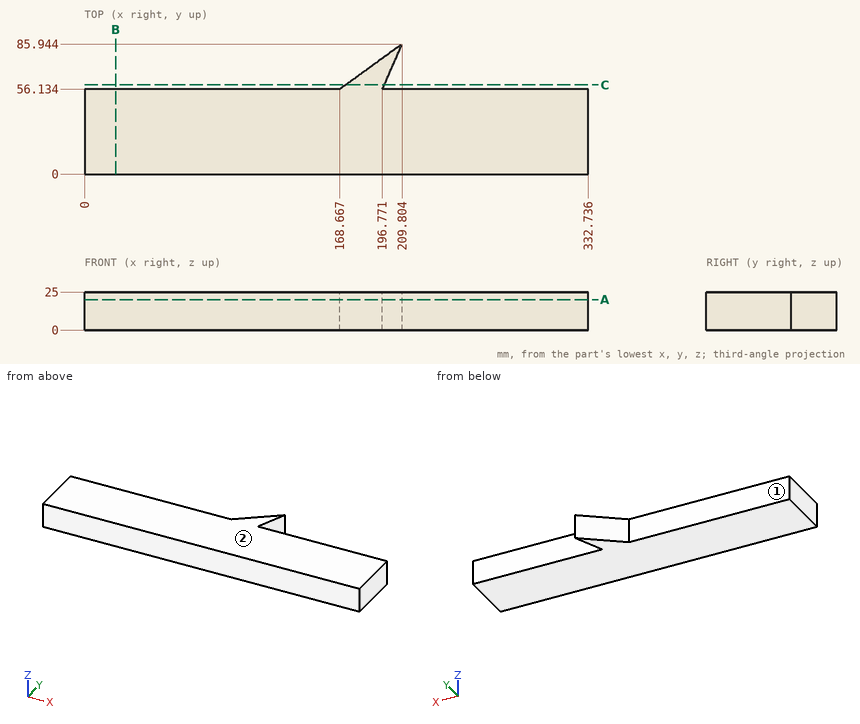
Design review of the part shown in the three views and the two pictorial views. Dimensions are in mm from the part's minimum x, y and z. A direction names the side the tool comes from. Give positions to 0.01 mm unless a question says otherwise; leave off trailing zeros. Loops run counter-clockwise (first coordinate to the right, second up) from the corner with the lowest first, then second, coordinate; pieces in that order, holes last. Notation, with made-up numbers: (86, 1) - (139, 1) arc R20 cw to (139, 9) - close; hole circle Ø2 at (-11.5, 86.25). An arc over 180 degrees is marked (long way). Answer as a JSON object with one key per item and string values.
Q1. Add section B-B on x = 20.5. State the section outline as (y, z) points (1 decimal).
Worked out:
{"outline": "(0, 0) - (56.1, 0) - (56.1, 25) - (0, 25) - close"}
Q2. Add section A-A on z = 20. State the section outline as (x, y) points (1 decimal), plus the area to 3 significant figures.
Worked out:
{"outline": "(0, 0) - (332.7, 0) - (332.7, 56.1) - (196.8, 56.1) - (209.8, 85.9) - (168.7, 56.1) - (0, 56.1) - close", "area": "19,100 mm^2"}
Q3. Add section C-C on y = 59. State the section outline as (x, z) points, plus the area to 3 significant figures.
Worked out:
{"outline": "(172.62, 0) - (198.02, 0) - (198.02, 25) - (172.62, 25) - close", "area": "635 mm^2"}
Q4. Insertion check: pin 1 (1.5 mm diameter, centred on x = 86, z = 7, fed in from +Y); pin 2 (6 mm diameter, centred on y = 73, z = 5, fed in from -X). Each pin has a flat end and moves straight along its axis. Give the tip position at first contact, or say it passes through.
Worked out:
{"pin 1": "stops at y = 56.13", "pin 2": "stops at x = 187.8"}
Q5. To check wall thickness, follow line 1 along Y through (x, z) = (36.5, 22) (1 decimal); line 2 along X through (y, z) = (74, 22.5) (1 decimal); line 3 along X through (y, z) = (81, 5) (1 decimal). State the ranges of each line that lie inside material, in increasing order.
Worked out:
{"line 1": "y = 0 to 56.1", "line 2": "x = 193.3 to 204.6", "line 3": "x = 203 to 207.6"}
Q6. For the marked faces 1 and 2, list the 3-axis set-ups (+Z, -Z, +X, -X, +Y, -Y) from which the entire face can be reached by the end or side of a thin tool; tool diameter is ignored.
Worked out:
{"face 1": "+Z, -Z, -X, +Y", "face 2": "+Z, +X, -X, +Y, -Y"}
